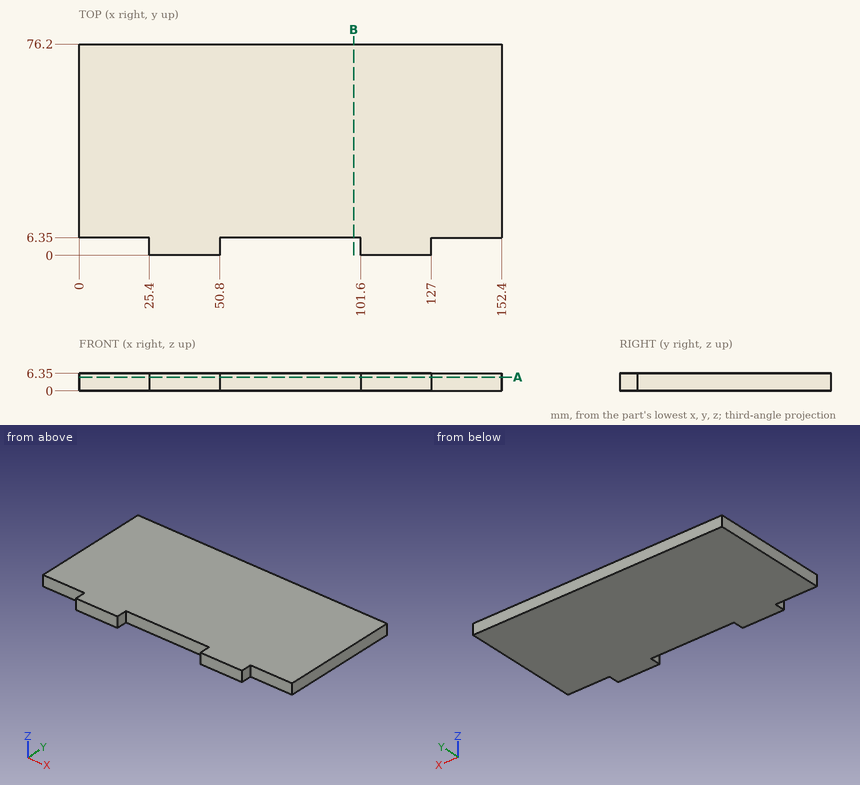
The figure shows three views and two pictorial views of one solid part (mm, origin at its lowest corner). Answer the questions. Give positions to 0.01 mm unless a question says otherwise; leave off trailing zeros. Write each loop counter-clockwise with the first axis right and the second up, starting at its lowest first coordinate (ties: lowest second). Pieces come first, ordered by that corner, then holes. Notation, with made-up numbers: (15.5, 14) -> (47.5, 14) arc R20 cw to (47.5, 18) -> close; hole circle Ø8 at (36, 34). An arc over 180 degrees is marked (long way). Write each question's results on one line, items separated by ' | '.
1. Straight lines are drawn through the part: L1, parallel to X at y = 5.5, z = 3.25; L2, parallel to Y at x = 70, z = 2.75. For each, find the intervals that lie inside material, in ascending order.
Data:
L1: 25.4 to 50.8, 101.6 to 127 | L2: 6.35 to 76.2
2. Each of these flat-tipped pins is pushed along its axis until it touches: pin 1 Ø3 at (x, z) = (83, 2.5) entering from -Y; pin 2 Ø3 at (y, z) = (2.5, 2.5) entering from -X; pin 3 Ø3 at (y, z) = (1.5, 4) entering from +X. Where does it stop, or does it pass through?
Data:
pin 1: y = 6.35 | pin 2: x = 25.4 | pin 3: x = 127
3. Find section A-A on z = 5. Determine the outline of the cut face in (x, y), and give its area (3 significant figures).
Data:
outline: (0, 6.35) -> (25.4, 6.35) -> (25.4, 0) -> (50.8, 0) -> (50.8, 6.35) -> (101.6, 6.35) -> (101.6, 0) -> (127, 0) -> (127, 6.35) -> (152.4, 6.35) -> (152.4, 76.2) -> (0, 76.2) -> close | area: 11,000 mm^2
4. Find section B-B on x = 99. Determine the outline of the cut face in (y, z), and give its area (3 significant figures).
Data:
outline: (6.35, 0) -> (76.2, 0) -> (76.2, 6.35) -> (6.35, 6.35) -> close | area: 444 mm^2
